Build history of the part. All positions in model axes, mm. A direction names the side the tool comes from. Give positions to 0.01 mm unless a question says otherwise; leave off trailing zeros. Order: outer loops, then holes, each group sorted by start corner. A loop starts at its lowest first (then second) coordinate and runs counter-clockwise, first axis right, second up. Notation, with made-up numbers: (79, -39.5) - (91, -39.5) arc R10 ccw to (91, -33.5) - close; hole circle Ø10 at (-27, 72.25). An arc over 180 degrees is marked (long way). Use a Markdown table: item, result.
Autodesk Inventor part; units mm, degrees
ref_plane "YZ Plane" through (0, 0, 0) normal (1, 0, 0) x (0, 1, 0)
ref_plane "XZ Plane" through (0, 0, 0) normal (0, 1, 0) x (-1, 0, 0)
ref_plane "XY Plane" through (0, 0, 0) normal (0, 0, 1) x (1, 0, 0)
sketch "Sketch1" plane through (0, 0, 0) normal (0, 0, 1) x (1, 0, 0)
  line L0 (42.5, -120) -> (-42.5, -120)
  line L1 (-42.5, -120) -> (-42.5, 120)
  line L2 (-42.5, 120) -> (42.5, 120)
  line L3 (42.5, 120) -> (42.5, -120)
  line L4 (42.5, -120) -> (-42.5, 120) construction
  line L5 (-42.5, -120) -> (42.5, 120) construction
  point P0 (0, 0)
  dimension "d42" = 85
  dimension "d43" = 240
extrude "Extrusion1" add sketch "Sketch1" against normal blind 12
sketch "Sketch2" plane through (0, 0, -12) normal (0, 0, -1) x (1, 0, 0)
  line L0 (42.5, -120) -> (42.5, 120)
  line L1 (0, -50) -> (0, 50)
  line L2 (0, -65) -> (0, -35) construction
  line L3 (9, -65) -> (9, -35)
  line L4 (-9, -35) -> (-9, -65)
  arc A0 (-9, -65) -> (9, -65) centre (0, -65) ccw
  arc A1 (9, -35) -> (-9, -35) centre (0, -35) ccw
  line L5 (0, 35) -> (0, 65) construction
  line L6 (9, 35) -> (9, 65)
  line L7 (-9, 65) -> (-9, 35)
  arc A2 (-9, 35) -> (9, 35) centre (0, 35) ccw
  arc A3 (9, 65) -> (-9, 65) centre (0, 65) ccw
  point P0 (0, 0)
  point P1 (0, -50)
  point P2 (0, 0)
  dimension "d46" = 100
  dimension "d47" = 30
  dimension "d48" = 18
  dimension "d49" = 30
  dimension "d50" = 18
extrude "Extrusion2" cut sketch "Sketch2" against normal through all
equation "\"d49\" = d47"
equation "\"d50\" = d48"
properties part number "StairsConnectionPlate" material "Steel"
1) Two-plate mould, pull along Y, no slides. Class faces 1 (the flat face through (1, -120, -6)), 2 (the flat face through (-9, -50, -6)), 3 (the flat face through (-1, 120, -6)), 4 (the flat face through (42.5, 2, -6)): +Y half, -Y half, draft (parallel to the pull), parting line (faces both ways), or undercut.
Computed:
| item | result |
|---|---|
| face 1 | -Y half |
| face 2 | undercut |
| face 3 | +Y half |
| face 4 | draft |
2) Wall check: line 1 (X direction, y = -48, z = -6.5); line 2 (Y direction, x = 7.5, z = -7); line 3 (Y direction, x = -1.5, z = -0.75). Give the ranges that are in metal, low to high. Write a range as from..to.
Computed:
| item | result |
|---|---|
| line 1 | x = -42.5..-9, 9..42.5 |
| line 2 | y = -120..-69.97, -30.03..30.03, 69.97..120 |
| line 3 | y = -120..-73.87, -26.13..26.13, 73.87..120 |
3) Tool access for faces 5 (the flat face through (-1, 2, 0)), 6 (the cylindrical face through (0, 26, -6)): list every direction of +Z, -Z, +X, -X, +Y, -Y with a clear straight run to the whole face (end or side of a thin tool).
Computed:
| item | result |
|---|---|
| face 5 | +Z, +X, -X, +Y, -Y |
| face 6 | +Z, -Z |
4) Slice it at B-B (y = 38.5). Write the cut outline in (x, z).
Computed:
| item | result |
|---|---|
| outline | (-42.5, -12) - (-9, -12) - (-9, 0) - (-42.5, 0) - close; (9, -12) - (42.5, -12) - (42.5, 0) - (9, 0) - close |
5) Slice it at C-C (z = -8.5). Write the cut outline in (x, y), and give its area (3 significant figures).
Computed:
| item | result |
|---|---|
| outline | (-42.5, -120) - (42.5, -120) - (42.5, 120) - (-42.5, 120) - close; hole (-9, -65) arc R9 ccw to (9, -65) - (9, -35) arc R9 ccw to (-9, -35) - close; hole (-9, 35) arc R9 ccw to (9, 35) - (9, 65) arc R9 ccw to (-9, 65) - close |
| area | 18,800 mm² |
6) Slice it at A-A (x = 0). Write the cut outline in (y, z), and give its area (3 significant figures).
Computed:
| item | result |
|---|---|
| outline | (-120, -12) - (-74, -12) - (-74, 0) - (-120, 0) - close; (-26, -12) - (26, -12) - (26, 0) - (-26, 0) - close; (74, -12) - (120, -12) - (120, 0) - (74, 0) - close |
| area | 1,730 mm² |
7) Pin check, flat tip, straight feed: P1, Ø2, axis at x = 5, y = -19, coming from the +Z side. Stop position of the tip, or through.
Computed:
| item | result |
|---|---|
| P1 | stops at z = 0 |
